```python
from build123d import *

# Parameters (mm, degrees)
F0_R     = 1.5
F0_R_2   = 6.5
F1_DEPTH = 25
F0_R_3   = 2.5
F2_DEPTH = 35
F3_DEPTH = 45


# Not quite as in the source:
# - a feature names something its author has since deleted; it is built from what else it names


with BuildPart() as f1:
    # F0 (on Top) → F1 (new body)
    with BuildSketch(Plane.XY):
        Polygon((15.5, 21), (-15.5, 21), (-21, 15.5), (-21, -15.5), (-15.5, -21), (15.5, -21), (21, -15.5), (21, 15.5), align=None)
        with Locations((-15.5, -15.5)):
            Circle(F0_R, mode=Mode.SUBTRACT)
        with Locations((15.5, -15.5)):
            Circle(F0_R, mode=Mode.SUBTRACT)
        with Locations((-15.5, 15.5)):
            Circle(F0_R, mode=Mode.SUBTRACT)
        Circle(F0_R_2, mode=Mode.SUBTRACT)
        with Locations((15.5, 15.5)):
            Circle(F0_R, mode=Mode.SUBTRACT)
    extrude(amount=F1_DEPTH)

    # F0 (on Top) → F2 (join)
    with BuildSketch(Plane.XY):
        Circle(F0_R_2)
        Circle(F0_R_3, mode=Mode.SUBTRACT)
    extrude(amount=F2_DEPTH)

    # F0 (on Top) → F3 (join)
    with BuildSketch(Plane.XY):
        Circle(F0_R_3)
    extrude(amount=F3_DEPTH)


solid = f1.part
```
Geometry check sheet. Reference: the model listing, model coordinates, mm. A direction names the side the tool comes from. Give positions to 0.01 mm unless a question says otherwise; leave off trailing zeros. Loops run counter-clockwise (first coordinate to the right, second up) from the corner with the lowest first, then second, coordinate; pieces in that order, holes last. Notation, with made-up numbers: M -22.5,24 L 32.5,24 A20 cw 32.5,39 Z; hole C 33.25,-28 d1. An arc over 180 degrees is marked long. Write item = value, one per line.
(1) Gauge pin test, flat ends, axial feed: pin 1 Ø2.5 at (x, y) = (-15.5, 15.5) entering from -Z; pin 2 Ø8 at (x, y) = (5, -15.5) entering from +Z. Record the tip position at first contact, or that the pin passes through.
Answer below:
pin_1 = through
pin_2 = 25
(2) Release check for a two-part mould opening along Y. For faces 3 (the face through (14, -15.43, 12.32)), 4 (the face through (18.3, 18.2, 12.3)), 5 (the face through (-17, 15.57, 12.32)), 6 (the face through (-18.3, -18.2, 12.3)) record: released by +Y, released by -Y, zero draft, split by the parting line, or undercut.
Answer below:
face_3 = undercut
face_4 = released by +Y
face_5 = undercut
face_6 = released by -Y
(3) Tool access check on faces 1 (the face through (-0.54, -2.44, 39.93)), 2 (the face through (14, 15.57, 12.32)). Record the directions out of +Z, -Z, +X, -X, +Y, -Y that give a thin tool (end or side, any length) a straight path to the whole face; none if there is none.
Answer below:
face_1 = +Z
face_2 = +Z, -Z
(4) Sectioned sample at A-A, the plane z = 22. Record the cut outline in (x, y).
Answer below:
outline = M -21,-15.5 L -15.5,-21 L 15.5,-21 L 21,-15.5 L 21,15.5 L 15.5,21 L -15.5,21 L -21,15.5 Z; hole C -15.5,-15.5 d3; hole C -15.5,15.5 d3; hole C 15.5,-15.5 d3; hole C 15.5,15.5 d3
(5) Sectioned sample at D-D, the plane z = 27. Record the cut outline in (x, y), plus the area to 3 significant figures.
Answer below:
outline = C 0,0 d13
area = 133 mm2
(6) Material ranges on line 1 (Y direction, x = -15.5, z = 18.5); line 2 (X direction, y = -15, z = 15); line 3 (Z direction, x = 16, y = 11.5), recorded low to high. Write a range as [from, to].
Answer below:
line_1 = [-21, -17], [-14, 14], [17, 21]
line_2 = [-21, -16.91], [-14.09, 14.09], [16.91, 21]
line_3 = [0, 25]
(7) Sectioned sample at C-C, the plane y = 5.5. Record the cut outline in (x, z), plus the area to 3 significant figures.
Answer below:
outline = M -21,0 L 21,0 L 21,25 L 3.46,25 L 3.46,35 L -3.46,35 L -3.46,25 L -21,25 Z
area = 1,120 mm2
(8) Sectioned sample at B-B, the plane x = 0. Record the cut outline in (y, z), plus the area to 3 significant figures.
Answer below:
outline = M -21,0 L 21,0 L 21,25 L 6.5,25 L 6.5,35 L 2.5,35 L 2.5,45 L -2.5,45 L -2.5,35 L -6.5,35 L -6.5,25 L -21,25 Z
area = 1,230 mm2
